The drawing under review shows one solid part. Ordinate dimensions are in mm from its lowest x, y, z. Round coordinates to 2 decimals unless told otherwise and drop trailing zeros. Order: outer loops, then holes, each group sorted by start corner. A loop starts at its lowest first (then second) coordinate and runs counter-clockwise, first axis right, second up. Notation, with made-up numbers: (-20, 39) - (10, 39) arc R9 ccw to (10, 45) - close; hole circle Ø11 at (-8.5, 63). An arc over 180 degrees is marked (long way). Answer as a JSON object with one key per item and string values. Group by question number.
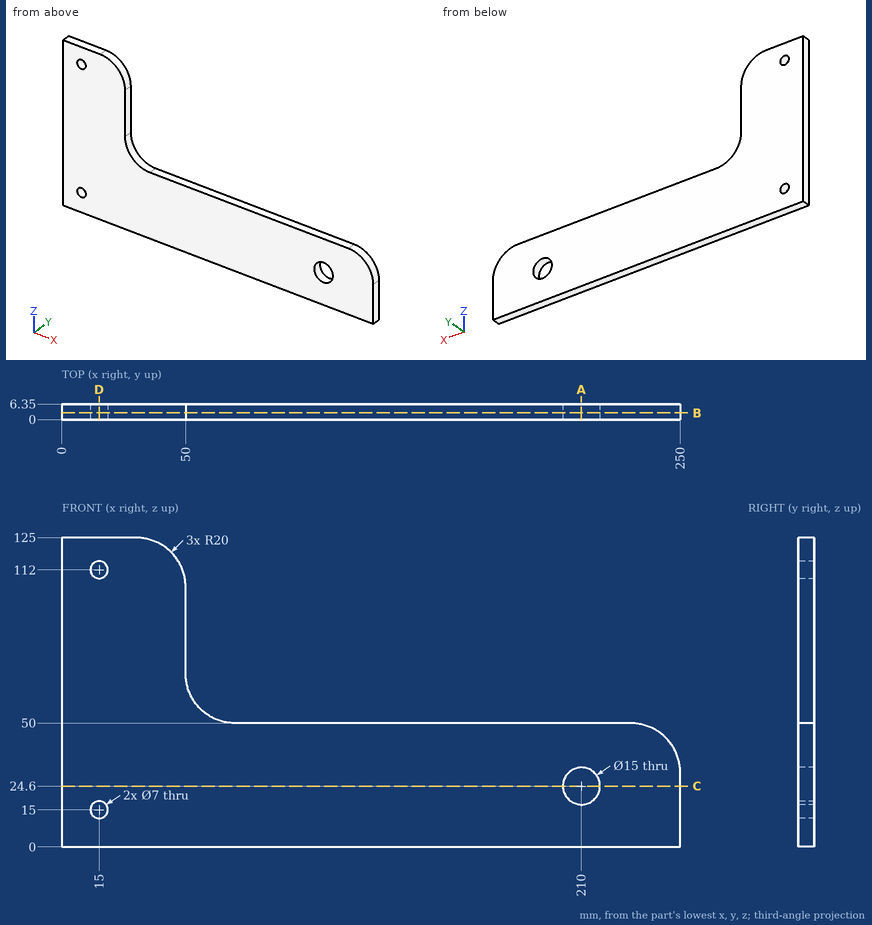
1. To check wall thickness, follow line 1 (Z direction, x = 15, y = 3.5); line 2 (X direction, y = 4.25, z = 24.6); line 3 (Z direction, x = 210, y = 3.75). State the ranges of each line that lie inside material, in increasing order. Write a range as from..to.
2. Take a section at D-D, the plane x = 15. Give the boundary of the cut face in (y, z).
3. Take a section at B-B, the plane y = 2.75. Give the boundary of the cut face in (x, z), then the cut area to 3 significant figures.
4. Clearance check with flat-ended pins moving along their axes: P1, Ø3, axis at y = 3, z = 84.5, coming from the +X side; P2, Ø3, axis at x = 119.5, y = 3, coming from the +Z side. State where each tip first meets the part, or that it passes through.
5. Take a section at A-A, the plane x = 210. Give the boundary of the cut face in (y, z), then the cut area to 3 significant figures.
6. Take a section at C-C, the plane z = 24.6. Give the boundary of the cut face in (x, y).
Response values:
{
 "1": {"line 1": "0..11.5, 18.5..108.5, 115.5..125", "line 2": "0..202.5, 217.5..250", "line 3": "0..17.1, 32.1..50"},
 "2": {"outline": "(0, 0) - (6.35, 0) - (6.35, 11.5) - (0, 11.5) - close; (0, 18.5) - (6.35, 18.5) - (6.35, 108.5) - (0, 108.5) - close; (0, 115.5) - (6.35, 115.5) - (6.35, 125) - (0, 125) - close"},
 "3": {"outline": "(0, 0) - (250, 0) - (250, 30) arc R20 ccw to (230, 50) - (70, 50) arc R20 cw to (50, 70) - (50, 105) arc R20 ccw to (30, 125) - (0, 125) - close; hole circle Ø7 at (15, 15); hole circle Ø7 at (15, 112); hole circle Ø15 at (210, 24.6)", "area": "15,900 mm2"},
 "4": {"P1": "x = 50", "P2": "z = 50"},
 "5": {"outline": "(0, 0) - (6.35, 0) - (6.35, 17.1) - (0, 17.1) - close; (0, 32.1) - (6.35, 32.1) - (6.35, 50) - (0, 50) - close", "area": "222 mm2"},
 "6": {"outline": "(0, 0) - (202.5, 0) - (202.5, 6.35) - (0, 6.35) - close; (217.5, 0) - (250, 0) - (250, 6.35) - (217.5, 6.35) - close"}
}
